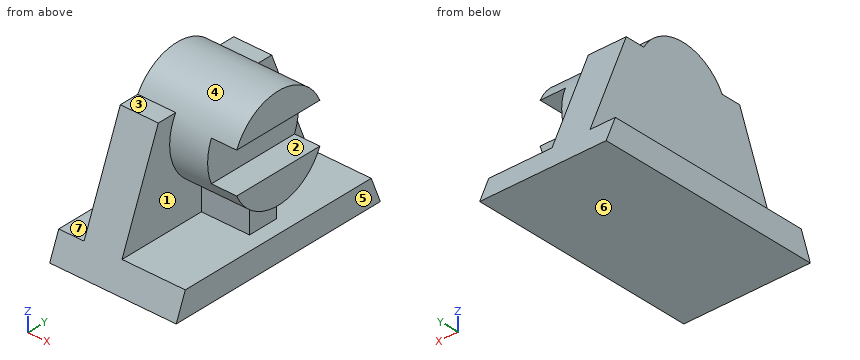
from build123d import *

# Parameters (mm, degrees)
F1_DEPTH      = 50
F2_W          = 25
F2_H          = 40
F2_W_2        = 10
F3_DEPTH      = 45.001
F3_DEPTH_BACK = 45.001
F4_R          = 20
F5_DEPTH      = 40
F6_W          = 12
F6_H          = 12
F7_DEPTH      = 19
F8_W          = 40
F8_H          = 16
F9_DEPTH      = 10


with BuildPart() as f1:
    # F0 (on Right) → F1 (new body)
    with BuildSketch(Plane.YZ):
        Polygon((-45, 0), (0, 0), (45, 0), (25, 50), (0, 50), (-25, 50), align=None)
    extrude(amount=-F1_DEPTH)

    # F2 (on Front) → F3 (cut, two sides)
    with BuildSketch(Plane.XZ) as f3_sk:
        with Locations((-12.5, 30)):
            Rectangle(F2_W, F2_H)
        with Locations((-45, 30)):
            Rectangle(F2_W_2, F2_H)
    extrude(amount=-F3_DEPTH, mode=Mode.SUBTRACT)
    extrude(f3_sk.sketch, amount=F3_DEPTH_BACK, mode=Mode.SUBTRACT)

    # F4 (on face) → F5 (join)
    with BuildSketch(Plane(origin=(-40, 0, 0), x_dir=(0, -1, 0), z_dir=(-1, 0, 0))):
        with Locations((0, 40)):
            Circle(F4_R)
    extrude(amount=-F5_DEPTH)

    # F6 (on face) → F7 (join)
    with BuildSketch(Plane.YZ.offset(-25)):
        with Locations((0, 16)):
            Rectangle(F6_W, F6_H)
    extrude(amount=F7_DEPTH)

    # F8 (on face) → F9 (cut)
    with BuildSketch(Plane.YZ):
        with Locations((0, 40)):
            Rectangle(F8_W, F8_H)
    extrude(amount=-F9_DEPTH, mode=Mode.SUBTRACT)


solid = f1.part
Design review of the part built by this model. Coordinates are the model's own, in mm. Face numbers are marked on the shaded views. A direction names the side the tool comes from. Give positions to 0.01 mm unless a question says otherwise; leave off trailing zeros. Write each loop counter-clockwise with the first axis right and the second up, starting at its lowest first coordinate (ties: lowest second). Pieces come first, ordered by that corner, then holes. Notation, with made-up numbers: M 41.25,-7.5 L 98.25,-7.5 A24 cw 98.25,21.5 Z; hole C 37.5,23.5 d4. An arc over 180 degrees is marked long. Answer as a JSON object with one key per item and string values. Group by question number.
1) We need section D-D (x = -11). Give the boundary of the cut face in (y, z).
2) We need section A-A (x = -5). Give the boundary of the cut face in (y, z).
3) Clearance check with flat-ended pins moving along their axes: pin 1 Ø7.5 at (x, y) = (-16, 14) entering from +Z; pin 2 Ø2 at (x, z) = (-26.5, 36) entering from -Y; pin 3 Ø4 at (x, y) = (-31.5, 20) entering from +Z. State where each tip first meets the part, or that it passes through.
4) Tool access review of the marked faces 1, 2 and 3: name each direction out of +Z, -Z, +X, -X, +Y, -Y from which nothing blocks a thin tool from reaching the whole face with its end or side.
5) We need section B-B (z = 40). Give the boundary of the cut face in (x, y).
6) Mouldability with a two-part tool opening along Z and no side actions: class the marked faces 4, 5, 6 and 7 as released by +Z, released by -Z, zero draft, split by the parting line, or undercut.
7) We need section C-C (y = 0). Give the boundary of the cut face in (x, z).
8) For line 1 along X through (y, z) = (-23, 27); line 2 along Z through (x, y) = (-7, 5); line 3 along X through (y, z) = (-14, 44), list the stretches that pass through material, from the lowest coordinate up.
Answer key:
{
 "1": {"outline": "M -45,0 L 45,0 L 41,10 L 6,10 L 6,20.92 A20 ccw long -6,20.92 L -6,10 L -41,10 Z"},
 "2": {"outline": "M -45,0 L 45,0 L 41,10 L -41,10 Z; M -18.33,32 A20 ccw 18.33,32 Z; M -18.33,48 L 18.33,48 A20 ccw Z"},
 "3": {"pin 1": "stops at z = 57.17", "pin 2": "stops at y = -31", "pin 3": "stops at z = 50"},
 "4": {"face 1": "+X, -Y", "face 2": "+X, +Y, -Y", "face 3": "+Z, +X, -X, -Y"},
 "5": {"outline": "M -40,-29 L -25,-29 L -25,-20 L -10,-20 L -10,20 L -25,20 L -25,29 L -40,29 Z"},
 "6": {"face 4": "undercut", "face 5": "zero draft", "face 6": "released by -Z", "face 7": "released by +Z"},
 "7": {"outline": "M -50,0 L 0,0 L 0,10 L -6,10 L -6,20 L 0,20 L 0,32 L -10,32 L -10,48 L 0,48 L 0,60 L -40,60 L -40,10 L -50,10 Z"},
 "8": {"line 1": "x = -40 to -25", "line 2": "z = 0 to 32, 48 to 59.36", "line 3": "x = -40 to -10"}
}
